from build123d import *

# Parameters (mm, degrees)
F1_W     = 25.4
F1_H     = 25.4
F2_DEPTH = 381


# Not quite as in the source:
# - a feature of the source that left no trace in its solid (it failed there, or was rolled back) is left out


with BuildPart() as f2:
    # F1 (on Top) → F2 (new body)
    with BuildSketch(Plane.XY):
        with BuildLine():
            ThreePointArc((25.4, 19.05), (11.9296158184, 24.6296158184), (6.35, 38.1))
            Line((6.35, 38.1), (-6.35, 38.1))
            ThreePointArc((-6.35, 38.1), (-11.9296158184, 24.6296158184), (-25.4, 19.05))
            Line((-25.4, 19.05), (-25.4, -38.1))
            Line((-25.4, -38.1), (-12.7, -38.1))
            ThreePointArc((-12.7, -38.1), (0, -25.4), (12.7, -38.1))
            Line((12.7, -38.1), (25.4, -38.1))
            Line((25.4, -38.1), (25.4, 19.05))
        make_face()
        Rectangle(F1_W, F1_H, mode=Mode.SUBTRACT)
    extrude(amount=F2_DEPTH)


solid = f2.part
Could you check a few things on this model? Use its own coordinates, in mm. A direction names the side the tool comes from. Coordinates: 2 decimals unless noted, no trailing zeros. Order: outer loops, then holes, each group sorted by start corner. A loop starts at its lowest first (then second) coordinate and runs counter-clockwise, first axis right, second up.
Q1. Thinking about a two-plate mould opening in Y: for faces 3 (the cylindrical face through (-0.279, -25.403, 187.833)), 4 (the flat face through (12.7, 0, 188)), 5 (the flat face through (0, -12.7, 188)), 6 (the flat face through (0, 38.1, 188)), which applies, released by +Y, released by -Y, zero draft, split by the parting line, or undercut?
Q2. Please list where these lines run through material, in increasing order: L1, parallel to X at y = 5.5, z = 113; L2, parallel to Y at x = -0.5, z = 244; L3, parallel to Y at x = 9, z = 114.
Q3. Suppose I cut it at B-B on x = 0. Please give me the cut outline in (y, z).
Q4. Suppose I cut it at D-D on x = -22. Please give me the cut outline in (y, z), and give its area (3 significant figures).
Q5. Suppose I cut it at C-C on z = 161. Please give me the cut outline in (x, y).
Q6. Which directions (+Z, -Z, +X, -X, +Y, -Y) give clear straight access to the entire face, cutting with the end or side of a thin tool? Please do faces 1 (the flat face through (-12.7, 0, 188)), 2 (the flat face through (0, -16, 381)).
Q7. Suppose I cut it at A-A on y = 4.5. Please give me the cut outline in (x, z), and give its area (3 significant figures).
Q8. Will these pins go through, and if not, where does the flat tip stop? pin 1 (2 mm diameter, centred on x = -17, z = 224.5, fed in from +Y); pin 2 (1.5 mm diameter, centred on x = -12.5, z = 217, fed in from +Y); pin 3 (20.5 mm diameter, centred on x = 1, z = 134, fed in from -Y).
Answer:
1. face 3: released by -Y
1. face 4: undercut
1. face 5: undercut
1. face 6: released by +Y
2. L1: x = -25.4 to -12.7, 12.7 to 25.4
2. L2: y = -25.41 to -12.7, 12.7 to 38.1
2. L3: y = -29.14 to -12.7, 12.7 to 28.41
3. outline: (-25.4, 0) - (-12.7, 0) - (-12.7, 381) - (-25.4, 381) - close; (12.7, 0) - (38.1, 0) - (38.1, 381) - (12.7, 381) - close
4. outline: (-38.1, 0) - (19.36, 0) - (19.36, 381) - (-38.1, 381) - close
4. area: 21,900 mm2
5. outline: (-25.4, -38.1) - (-12.7, -38.1) arc R12.7 cw to (12.7, -38.1) - (25.4, -38.1) - (25.4, 19.05) arc R19.05 cw to (6.35, 38.1) - (-6.35, 38.1) arc R19.05 cw to (-25.4, 19.05) - close; hole (-12.7, -12.7) - (12.7, -12.7) - (12.7, 12.7) - (-12.7, 12.7) - close
6. face 1: +Z, -Z
6. face 2: +Z, +X, -X, +Y, -Y
7. outline: (-25.4, 0) - (-12.7, 0) - (-12.7, 381) - (-25.4, 381) - close; (12.7, 0) - (25.4, 0) - (25.4, 381) - (12.7, 381) - close
7. area: 9,680 mm2
8. pin 1: stops at y = 21.53
8. pin 2: stops at y = 24.81
8. pin 3: stops at y = -32.21
